Verification items for the finished model (mm, model axes). Face numbers are marked on the shaded views. A direction names the side the tool comes from. Coordinates: 2 decimals unless noted, no trailing zeros. Loops run counter-clockwise (first coordinate to the right, second up) from the corner with the lowest first, then second, coordinate; pieces in that order, holes last. Notation, with made-up numbers: (11, -2) -> (53, -2) arc R5 cw to (53, 4) -> close; hole circle Ø2 at (18.5, -39). An arc over 180 degrees is marked (long way). Answer as a JSON object with one key per item and string values. Group by question number.
Q1. Cross-section at C-C on z = 4.5. Record the boundary of the cut face in (x, y).
Q2. Cross-section at B-B on y = 9.5. Record the boundary of the cut face in (x, z).
Q3. Cross-section at D-D on x = 13.5. Record the boundary of the cut face in (y, z).
Q4. Set-up check for the marked faces 1 and 2: record each of +Z, -Z, +X, -X, +Y, -Y from which the full face is reachable in a straight line by a thin tool's end or side.
Q5. Scan lines: L1, parallel to X at y = 10.25, z = 20.5; L2, parallel to Z at x = 20.5, y = 9.5. Record each from-to range of solid material in increasing order.
Q6. Cross-section at A-A on x = 6.75. Record the boundary of the cut face in (y, z).
Q7. Release check for a two-part mould opening along Z. For the marked faces 3, 4, 5 and 6 record: released by +Z, released by -Z, zero draft, split by the parting line, or undercut.
Q8. Gauge pin test, flat end, axial feed: pin 1 Ø4 at (x, z) = (16, 6) entering from -Y. Record the tip position at first contact, or that the pin passes through.
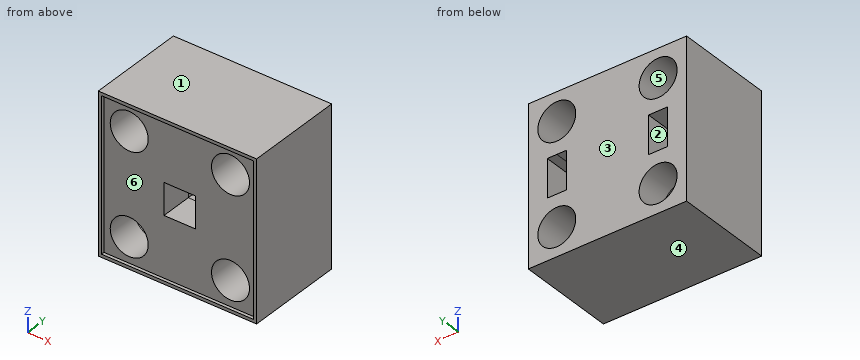
Autodesk Inventor part; units mm, degrees
ref_plane "YZ Plane" through (0, 0, 0) normal (1, 0, 0) x (0, 1, 0)
ref_plane "XZ Plane" through (0, 0, 0) normal (0, 1, 0) x (-1, 0, 0)
ref_plane "XY Plane" through (0, 0, 0) normal (0, 0, 1) x (1, 0, 0)
sketch "Sketch1" plane through (0, 0, 0) normal (0, 1, 0) x (-1, 0, 0)
  line L0 (0, 0) -> (-25, 0)
  line L1 (-25, 0) -> (-25, 25)
  line L2 (-25, 25) -> (0, 25)
  line L3 (0, 25) -> (0, 0)
  line L4 (-10, 12.5) -> (-10, 15)
  line L5 (-10, 15) -> (-12.5, 15)
  line L6 (-10, 12.5) -> (-10, 10)
  line L7 (-10, 10) -> (-12.5, 10)
  line L8 (-15, 12.5) -> (-15, 15)
  line L9 (-15, 15) -> (-12.5, 15)
  line L10 (-15, 12.5) -> (-15, 10)
  line L11 (-15, 10) -> (-12.5, 10)
  circle A0 centre (-4.5, 4.5) radius 3
  circle A1 centre (-20.5, 20.5) radius 3
  circle A2 centre (-4.5, 20.5) radius 3
  circle A3 centre (-20.5, 4.5) radius 3
  dimension "d0" = 25
  dimension "d1" = 25
  dimension "d2" = 2.5
  dimension "d3" = 2.5
  dimension "d4" = 2.5
  dimension "d5" = 2.5
  dimension "d6" = 2.5
  dimension "d8" = 6
  dimension "d9" = 6
  dimension "d10" = 6
  dimension "d11" = 6
extrude "Extrusion1" add sketch "Sketch1" along normal blind 5
sketch "Sketch4" plane through (0, 0, 0) normal (0, -1, 0) x (1, 0, 0)
  line L0 (0, 0) -> (0, 25)
  line L1 (25, 25) -> (25, 0)
  line L2 (0, 25) -> (25, 25)
  line L3 (25, 25) -> (25, 0)
  line L4 (25, 0) -> (0, 0)
  line L5 (0, 0) -> (0, 25)
  line L6 (0.5, 24.5) -> (24.5, 24.5)
  line L7 (24.5, 24.5) -> (24.5, 0.5)
  line L8 (24.5, 0.5) -> (0.5, 0.5)
  line L9 (0.5, 0.5) -> (0.5, 24.5)
  dimension "d18" = 24
  dimension "d19" = 24
extrude "Extrusion3" add sketch "Sketch4" along normal blind 0.5
sketch "Sketch5" plane through (0, 5, 0) normal (0, 1, 0) x (1, 0, 0)
  line L0 (20.5, -15.5) -> (17, -15.5)
  line L1 (17, -15.5) -> (17, -9.5)
  line L2 (17, -9.5) -> (20.5, -9.5)
  line L3 (20.5, -15.5) -> (24, -15.5)
  line L4 (24, -15.5) -> (24, -9.5)
  line L5 (24, -9.5) -> (20.5, -9.5)
  line L6 (8, -15.5) -> (4.5, -15.5)
  line L7 (4.5, -9.5) -> (8, -9.5)
  line L8 (8, -9.5) -> (8, -15.5)
  line L9 (4.5, -15.5) -> (1, -15.5)
  line L10 (1, -15.5) -> (1, -9.5)
  line L11 (1, -9.5) -> (4.5, -9.5)
  circle A0 centre (20.5, -20.5) radius 3
  circle A1 centre (4.5, -20.5) radius 3
  circle A2 centre (20.5, -4.5) radius 3
  circle A3 centre (4.5, -4.5) radius 3
  line L12 (15, -15) -> (10, -15)
  line L13 (10, -10) -> (15, -10)
  line L14 (15, -15) -> (10, -15)
  line L15 (10, -15) -> (10, -10)
  line L16 (10, -10) -> (15, -10)
  line L17 (15, -10) -> (15, -15)
  line L18 (25, -25) -> (0, -25)
  line L19 (25, -25) -> (0, -25)
  line L20 (0, -25) -> (0, 0)
  line L21 (0, 0) -> (25, 0)
  line L22 (25, 0) -> (25, -25)
  dimension "d22" = 3.5
  dimension "d23" = 6
  dimension "d24" = 3.5
  dimension "d25" = 3.5
  dimension "d26" = 6
  dimension "d27" = 3.5
  dimension "d28" = 6
  dimension "d29" = 6
  dimension "d30" = 6
  dimension "d31" = 6
extrude "Extrusion4" add sketch "Sketch5" along normal blind 5
sketch "Sketch6" plane through (0, 10, 0) normal (0, 1, 0) x (1, 0, 0)
  line L0 (17, -15.5) -> (24, -15.5)
  line L1 (17, -9.5) -> (24, -9.5)
  line L2 (20.5, -15.5) -> (22, -15.5)
  line L3 (22, -15.5) -> (22, -9.5)
  line L4 (22, -9.5) -> (20.5, -9.5)
  line L5 (20.5, -15.5) -> (19, -15.5)
  line L6 (19, -15.5) -> (19, -9.5)
  line L7 (19, -9.5) -> (20.5, -9.5)
  line L8 (8, -15.5) -> (1, -15.5)
  line L9 (8, -9.5) -> (1, -9.5)
  line L10 (4.5, -15.5) -> (6, -15.5)
  line L11 (6, -15.5) -> (6, -9.5)
  line L12 (6, -9.5) -> (4.5, -9.5)
  line L13 (4.5, -15.5) -> (3, -15.5)
  line L14 (3, -15.5) -> (3, -9.5)
  line L15 (3, -9.5) -> (4.5, -9.5)
  line L16 (25, -25) -> (0, -25)
  line L17 (25, -25) -> (0, -25)
  line L18 (0, -25) -> (0, 0)
  line L19 (0, 0) -> (25, 0)
  line L20 (25, 0) -> (25, -25)
  circle A0 centre (4.5, -20.5) radius 3
  circle A1 centre (20.5, -20.5) radius 3
  circle A2 centre (20.5, -4.5) radius 3
  circle A3 centre (4.5, -4.5) radius 3
  dimension "d34" = 1.5
  dimension "d35" = 1.5
  dimension "d36" = 1.5
  dimension "d37" = 1.5
  dimension "d38" = 6
  dimension "d39" = 6
  dimension "d40" = 6
  dimension "d41" = 6
extrude "Extrusion5" add sketch "Sketch6" along normal blind 5
properties part number "SiPM cover"
Computed values:
{
 "1": {"outline": "(0, -0.5) -> (0.5, -0.5) -> (0.5, 0) -> (1.5, 0) -> (1.5, 15) -> (0, 15) -> close; (7.5, 0) -> (17.5, 0) -> (17.5, 15) -> (7.5, 15) -> close; (23.5, 0) -> (24.5, 0) -> (24.5, -0.5) -> (25, -0.5) -> (25, 15) -> (23.5, 15) -> close"},
 "2": {"outline": "(0, 0) -> (25, 0) -> (25, 25) -> (0, 25) -> close; hole (1, 9.5) -> (8, 9.5) -> (8, 15.5) -> (1, 15.5) -> close; hole circle Ø6 at (4.5, 4.5); hole circle Ø6 at (4.5, 20.5); hole (10, 10) -> (15, 10) -> (15, 15) -> (10, 15) -> close; hole (17, 9.5) -> (24, 9.5) -> (24, 15.5) -> (17, 15.5) -> close; hole circle Ø6 at (20.5, 4.5); hole circle Ø6 at (20.5, 20.5)"},
 "3": {"outline": "(-0.5, 0) -> (15, 0) -> (15, 25) -> (-0.5, 25) -> (-0.5, 24.5) -> (0, 24.5) -> (0, 15) -> (10, 15) -> (10, 10) -> (0, 10) -> (0, 0.5) -> (-0.5, 0.5) -> close"},
 "4": {"face 1": "+Z, +X, -X, +Y, -Y", "face 2": "+Y"},
 "5": {"L1": "x = 0 to 1.5, 7.5 to 17.5, 23.5 to 25", "L2": "z = 0 to 1.5, 7.5 to 9.5, 15.5 to 17.5, 23.5 to 25"},
 "6": {"outline": "(-0.5, 0) -> (15, 0) -> (15, 2.52) -> (0, 2.52) -> (0, 0.5) -> (-0.5, 0.5) -> close; (-0.5, 24.5) -> (0, 24.5) -> (0, 22.48) -> (15, 22.48) -> (15, 25) -> (-0.5, 25) -> close; (0, 6.48) -> (15, 6.48) -> (15, 18.52) -> (0, 18.52) -> close; hole (5, 9.5) -> (10, 9.5) -> (10, 15.5) -> (5, 15.5) -> close"},
 "7": {"face 3": "zero draft", "face 4": "released by -Z", "face 5": "undercut", "face 6": "undercut"},
 "8": {"pin 1": "stops at y = 0"}
}
